Can you work these out from the model? Positions are in its coordinate system, mm. Face numbers are marked on the shaded views. A direction names the side the tool comes from. Round coordinates to 2 decimals unless told otherwise and drop trailing zeros. Order: outer loops, then holes, each group sorted by start corner. A loop starts at its lowest first (then second) coordinate and runs counter-clockwise, first axis right, second up. Notation, with made-up numbers: (42, 57.5) -> (98, 57.5) arc R19 cw to (98, 87.5) -> close; hole circle Ø1 at (17.5, -22). An arc over 180 degrees is marked (long way). One line per item, written item: value.
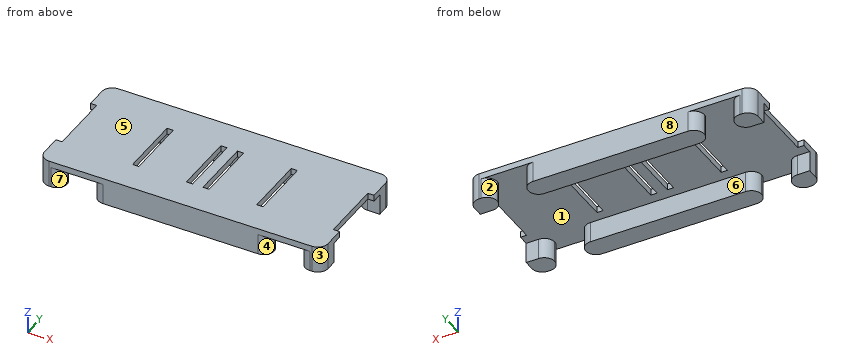
```python
from build123d import *

# Parameters (mm, degrees)
F0_W     = 150
F0_H     = 60
F1_DEPTH = 3
F2_W     = 3
F2_H     = 30
F3_DEPTH = 25
F4_W     = 6.5
F4_H     = 60
F5_DEPTH = 25
F6_W     = 85
F6_H     = 10
F6_W_2   = 11
F7_DEPTH = 10
F8_R     = 4.99999


# Not quite as in the source:
# - a fillet or chamfer is up to 0.001 mm smaller than in the source, because OpenCascade refuses the exact size


with BuildPart() as f1:
    # F0 (on Top) → F1 (new body)
    with BuildSketch(Plane.XY):
        Rectangle(F0_W, F0_H)
    extrude(amount=F1_DEPTH)

    # F2 (on Top) → F3 (cut)
    with BuildSketch(Plane.XY):
        with Locations((-4, 0)):
            Rectangle(F2_W, F2_H)
        with Locations((4, 0)):
            Rectangle(F2_W, F2_H)
        with Locations((67, 0)):
            Rectangle(F2_W, F2_H)
        with Locations((-67, 0)):
            Rectangle(F2_W, F2_H)
        with Locations((-30, 0)):
            Rectangle(F2_W, F2_H)
        with Locations((30, 0)):
            Rectangle(F2_W, F2_H)
    extrude(amount=F3_DEPTH, mode=Mode.SUBTRACT)

    # F4 (on Top) → F5 (cut)
    with BuildSketch(Plane.XY):
        with Locations((71.75, 0)):
            Rectangle(F4_W, F4_H)
        with Locations((-71.75, 0)):
            Rectangle(F4_W, F4_H)
    extrude(amount=F5_DEPTH, mode=Mode.SUBTRACT)

    # F6 (on Top) → F7 (join)
    with BuildSketch(Plane.XY):
        with Locations((0, 25)):
            Rectangle(F6_W, F6_H)
        with Locations((0, -25)):
            Rectangle(F6_W, F6_H)
        with Locations((63, 25)):
            Rectangle(F6_W_2, F6_H)
        with Locations((63, -25)):
            Rectangle(F6_W_2, F6_H)
        with Locations((-63, -25)):
            Rectangle(F6_W_2, F6_H)
        with Locations((-63, 25)):
            Rectangle(F6_W_2, F6_H)
    extrude(amount=-F7_DEPTH)

    # F8 (radius 5 in the source; OpenCascade refuses exactly that, so slightly less here)
    f8_edges = [f1.edges().sort_by_distance(p)[0] for p in [
        (-68.5, -30, -3.5),
        (-68.5, 30, -3.5),
        (68.5, 30, -3.5),
        (68.5, -30, -3.5),
        (42.5, 30, -5),
        (42.5, 20, -5),
        (42.5, -20, -5),
        (42.5, -30, -5),
        (57.5, 30, -5),
        (57.5, 20, -5),
        (57.5, -20, -5),
        (57.5, -30, -5),
        (-42.5, 30, -5),
        (-42.5, 20, -5),
        (-42.5, -20, -5),
        (-42.5, -30, -5),
        (-57.5, 30, -5),
        (-57.5, 20, -5),
        (-57.5, -20, -5),
        (-57.5, -30, -5),
    ]]
    fillet(f8_edges, radius=F8_R)


solid = f1.part
```
Q1. I want a section at A-A on y = -8. List the corners of the cut face in (x, z) for me.
Answers below:
outline: (-65.5, 0) -> (-31.5, 0) -> (-31.5, 3) -> (-65.5, 3) -> close; (-28.5, 0) -> (-5.5, 0) -> (-5.5, 3) -> (-28.5, 3) -> close; (-2.5, 0) -> (2.5, 0) -> (2.5, 3) -> (-2.5, 3) -> close; (5.5, 0) -> (28.5, 0) -> (28.5, 3) -> (5.5, 3) -> close; (31.5, 0) -> (65.5, 0) -> (65.5, 3) -> (31.5, 3) -> close
Q2. I want a section at C-C on z = -1.25. Give the number of separate pieces and of enclosed holes in the cut face, plus the area to 3 significant figures.
Answers below:
separate pieces: 6
enclosed holes: 0
area: 2,030 mm^2
Q3. Please list where these lines run through material, in increasing order: line 1 along Y through (x, z) = (-33.5, -3); line 2 along X through (y, z) = (-7.5, 2.25); line 3 along Z through (x, y) = (-49.5, -22).
Answers below:
line 1: -30 to -20, 20 to 30
line 2: -65.5 to -31.5, -28.5 to -5.5, -2.5 to 2.5, 5.5 to 28.5, 31.5 to 65.5
line 3: 0 to 3
Q4. We'd pull the mould along Y, two halves only. Please class the marked faces 6, 7 and 8: released by +Y, released by -Y, zero draft, split by the parting line, or undercut.
Answers below:
face 6: undercut
face 7: released by -Y
face 8: released by +Y
Q5. On a 3-axis mill with a long thin cutter (end or side, diameter ignored), from which of +Z, -Z, +X, -X, +Y, -Y can I reach the whole of each face in a straight line? I mean the marked faces 1, 2, 3, 4 and 5. Say none if no direction works.
Answers below:
face 1: -Z
face 2: -Z, +Y
face 3: +Z, -Z, +X, -Y
face 4: -Z, -Y
face 5: +Z, +X, -X, +Y, -Y
Q6. Will these pins go through, and if not, where does the flat tip stop? pin 1 Ø5 at (x, y) = (-54, -17) entering from -Z; pin 2 Ø1.5 at (y, z) = (-3, 1) entering from -X; pin 3 Ø5 at (x, z) = (67, -6.5) entering from +Y; pin 4 Ø2 at (y, z) = (-3, -1.5) entering from -X.
Answers below:
pin 1: z = 0
pin 2: x = -65.5
pin 3: y = 29.9
pin 4: through
Q7. I want a section at D-D on x = -40. List the corners of the cut face in (y, z) for me.
Answers below:
outline: (-30, 0) -> (-29.33, 0) -> (-29.33, -10) -> (-20.67, -10) -> (-20.67, 0) -> (20.67, 0) -> (20.67, -10) -> (29.33, -10) -> (29.33, 0) -> (30, 0) -> (30, 3) -> (-30, 3) -> close
Q8. I want a section at B-B on x = 22.5. List the corners of the cut face in (y, z) for me, plus the area to 3 significant figures.
Answers below:
outline: (-30, -10) -> (-20, -10) -> (-20, 0) -> (20, 0) -> (20, -10) -> (30, -10) -> (30, 3) -> (-30, 3) -> close
area: 380 mm^2
